Can you work these out from the model? Positions are in its coordinate system, mm. Face numbers are marked on the shaded views. A direction names the side the tool comes from. Give positions to 0.01 mm unless a question says otherwise; leave off trailing zeros. Loops run counter-clockwise (first coordinate to the right, second up) from the corner with the lowest first, then second, coordinate; pieces in that order, holes last. Notation, with made-up numbers: (35.5, 36) - (92.5, 36) arc R30 ccw to (92.5, 60) - close; hole circle Ø8 at (-37.75, -11.5). An arc over 180 degrees is marked (long way). Use a Markdown table: item, result. Add a question column.
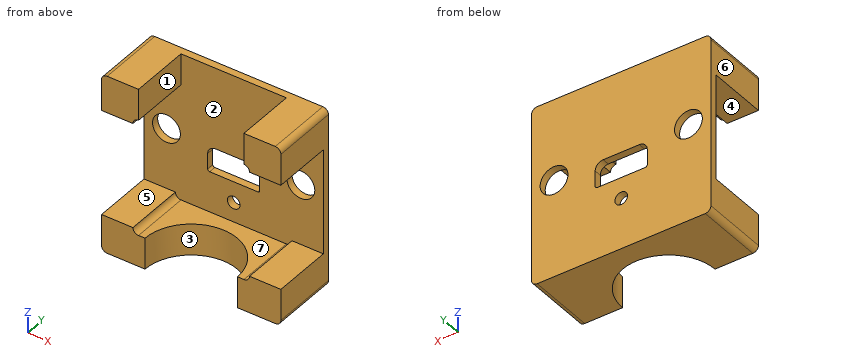
```python
from build123d import *

# Parameters (mm, degrees)
SKETCH2_R           = 1.575
BOSS_EXTRUDE3_DEPTH = 1.8
BOSS_EXTRUDE4_START = 15
BOSS_EXTRUDE4_DEPTH = 15
CUT_EXTRUDE1_REACH  = 54.232
SKETCH4_R           = 11.530245675
SKETCH5_R           = 3.475
CUT_EXTRUDE2_DEPTH  = 36.826264807


with BuildPart() as part:
    # Sketch2 → Boss-Extrude3 (new body)
    with BuildSketch(Plane(origin=(0, 0, 0), x_dir=(1, 0, 0), z_dir=(0, 1, 0))):
        with BuildLine():
            Line((-20.975, -22.375), (20.975, -22.375))
            ThreePointArc((20.975, -22.375), (21.964949494, -21.964949494), (22.375, -20.975))
            Line((22.375, -20.975), (22.375, 20.975))
            ThreePointArc((22.375, 20.975), (21.964949494, 21.964949494), (20.975, 22.375))
            Line((20.975, 22.375), (-20.975, 22.375))
            ThreePointArc((-20.975, 22.375), (-21.964949494, 21.964949494), (-22.375, 20.975))
            Line((-22.375, 20.975), (-22.375, -20.975))
            ThreePointArc((-22.375, -20.975), (-21.964949494, -21.964949494), (-20.975, -22.375))
        make_face()
        with Locations(Location((0, 9.655, 0), (0, 0, 270))):
            Circle(SKETCH2_R, mode=Mode.SUBTRACT)
        with BuildLine():
            Line((-4.5, -2), (4.5, -2))
            ThreePointArc((4.5, -2), (5.914213562, -1.414213562), (6.5, 0))
            Line((6.5, 0), (6.5, 3.9))
            ThreePointArc((6.5, 3.9), (6.353553391, 4.253553391), (6, 4.4))
            Line((6, 4.4), (-6, 4.4))
            ThreePointArc((-6, 4.4), (-6.353553391, 4.253553391), (-6.5, 3.9))
            Line((-6.5, 3.9), (-6.5, 0))
            ThreePointArc((-6.5, 0), (-5.914213562, -1.414213562), (-4.5, -2))
        make_face(mode=Mode.SUBTRACT)
    extrude(amount=BOSS_EXTRUDE3_DEPTH)

    # Sketch3 → Boss-Extrude4 (add)
    with BuildSketch(Plane.XZ.offset(BOSS_EXTRUDE4_START)):
        with BuildLine():
            Line((-20.975, -22.375), (20.975, -22.375))
            ThreePointArc((20.975, -22.375), (21.964949494, -21.964949494), (22.375, -20.975))
            Line((22.375, -20.975), (22.375, -13.15))
            Line((22.375, -13.15), (14.55, -13.15))
            ThreePointArc((14.55, -13.15), (14.139949494, -14.139949494), (13.15, -14.55))
            Line((13.15, -14.55), (-13.15, -14.55))
            ThreePointArc((-13.15, -14.55), (-14.139949494, -14.139949494), (-14.55, -13.15))
            Line((-14.55, -13.15), (-22.375, -13.15))
            Line((-22.375, -13.15), (-22.375, -20.975))
            ThreePointArc((-22.375, -20.975), (-21.964949494, -21.964949494), (-20.975, -22.375))
        make_face()
        with BuildLine():
            Line((-20.975, 22.375), (-13.15, 22.375))
            Line((-13.15, 22.375), (-13.15, 14.55))
            ThreePointArc((-13.15, 14.55), (-14.139949494, 14.139949494), (-14.55, 13.15))
            Line((-14.55, 13.15), (-22.375, 13.15))
            Line((-22.375, 13.15), (-22.375, 20.975))
            ThreePointArc((-22.375, 20.975), (-21.964949494, 21.964949494), (-20.975, 22.375))
        make_face()
        with BuildLine():
            Line((14.55, 13.15), (22.375, 13.15))
            Line((22.375, 13.15), (22.375, 20.975))
            ThreePointArc((22.375, 20.975), (21.964949494, 21.964949494), (20.975, 22.375))
            Line((20.975, 22.375), (13.15, 22.375))
            Line((13.15, 22.375), (13.15, 14.55))
            ThreePointArc((13.15, 14.55), (14.139949494, 14.139949494), (14.55, 13.15))
        make_face()
    extrude(amount=-BOSS_EXTRUDE4_DEPTH)

    # Sketch4 → Cut-Extrude1 (cut, up to next)
    with BuildSketch(Plane(origin=(0, 0, -22.375), x_dir=(-1, 0, 0), z_dir=(0, 0, -1)), mode=Mode.PRIVATE) as cut_extrude1_sk1:
        with Locations((0, -15)):
            Circle(SKETCH4_R)
    cut_extrude1_tool1 = extrude(cut_extrude1_sk1.sketch, amount=-CUT_EXTRUDE1_REACH, mode=Mode.PRIVATE) & part.part
    add(cut_extrude1_tool1.solids().sort_by_distance((0, -15, -22.375))[0], mode=Mode.SUBTRACT)

    # Sketch5 → Cut-Extrude2 (cut, through all)
    with BuildSketch(Plane(origin=(0, 1.8, 0), x_dir=(1, 0, 0), z_dir=(0, 1, 0))):
        with Locations(Location((-16.77, -1.975, 0), (0, 0, 270))):
            Circle(SKETCH5_R)
        with Locations(Location((16.77, -1.975, 0), (0, 0, 270))):
            Circle(SKETCH5_R)
    extrude(amount=-CUT_EXTRUDE2_DEPTH, mode=Mode.SUBTRACT)


solid = part.part
```
1. On a 3-axis mill with a long thin cutter (end or side, diameter ignored), from which of +Z, -Z, +X, -X, +Y, -Y can I reach the whole of each face in a straight line? I mean the marked faces 1, 2, 3 and 4. Say none if no direction works.
2. Suppose I cut it at C-C (y = -10.5). List the corners of the cut face in (x, z) for me (3 decimals), and give its area (3 significant figures).
3. Suppose I cut it at B-B (x = -16.77). List the corners of the cut face in (y, z) for me (3 decimals), and give its area (3 significant figures).
4. If we mould it in two halves opening along X, with no side actions, what happens to the marked faces 5, 6 and 7? For each: released by +X, released by -X, zero draft, split by the parting line, or undercut.
5. Please list where these lines run through material, in increasing order: line 1 along X through (y, z) = (-8.75, 20.5) (3 decimals); line 2 along Y through (x, z) = (-13, 3.5). Write a range as [from, to].
6. Suppose I cut it at D-D (z = 16.5). List the corners of the cut face in (x, y) for me (3 decimals).
7. Suppose I cut it at A-A (x = 0). List the corners of the cut face in (y, z) for me (3 decimals), and give its area (3 significant figures).
8. Will this pin go through, and if not, where does the flat tip stop? P1, Ø1, axis at x = -12, z = 3.5, coming from the -Y side.
Results below:
| question | item | result |
|---|---|---|
| 1 | face 1 | +Z, -Y |
| 1 | face 2 | -Y |
| 1 | face 3 | +Z, -Z, -Y |
| 1 | face 4 | +X, -X, -Y |
| 2 | outline | (-22.375, -20.975) arc R1.4 ccw to (-20.975, -22.375) - (-10.616, -22.375) - (-10.616, -14.55) - (-13.15, -14.55) arc R1.4 cw to (-14.55, -13.15) - (-22.375, -13.15) - close; (-22.375, 13.15) - (-14.55, 13.15) arc R1.4 cw to (-13.15, 14.55) - (-13.15, 22.375) - (-20.975, 22.375) arc R1.4 ccw to (-22.375, 20.975) - close; (10.616, -22.375) - (20.975, -22.375) arc R1.4 ccw to (22.375, -20.975) - (22.375, -13.15) - (14.55, -13.15) arc R1.4 cw to (13.15, -14.55) - (10.616, -14.55) - close; (13.15, 14.55) arc R1.4 cw to (14.55, 13.15) - (22.375, 13.15) - (22.375, 20.975) arc R1.4 ccw to (20.975, 22.375) - (13.15, 22.375) - close |
| 2 | area | 372 mm² |
| 3 | outline | (-15, -22.375) - (1.8, -22.375) - (1.8, -1.5) - (0, -1.5) - (0, -13.15) - (-15, -13.15) - close; (-15, 13.15) - (0, 13.15) - (0, 5.45) - (1.8, 5.45) - (1.8, 22.375) - (-15, 22.375) - close |
| 3 | area | 345 mm² |
| 4 | face 5 | zero draft |
| 4 | face 6 | released by -X |
| 4 | face 7 | undercut |
| 5 | line 1 | [-22.375, -13.15], [13.15, 22.375] |
| 5 | line 2 | [0, 1.8] |
| 6 | outline | (-22.375, -15) - (-13.15, -15) - (-13.15, 0) - (13.15, 0) - (13.15, -15) - (22.375, -15) - (22.375, 1.8) - (-22.375, 1.8) - close |
| 7 | outline | (-3.47, -22.375) - (1.8, -22.375) - (1.8, -11.23) - (0, -11.23) - (0, -14.55) - (-3.47, -14.55) - close; (0, -8.08) - (1.8, -8.08) - (1.8, -4.4) - (0, -4.4) - close; (0, 2) - (1.8, 2) - (1.8, 22.375) - (0, 22.375) - close |
| 7 | area | 90.5 mm² |
| 8 | P1 | y = 0 |
